The listing builds one solid part. Answer for the finished solid, in the listing's coordinates (mm). Round coordinates to 2 decimals unless told otherwise and drop trailing zeros. Write each loop counter-clockwise with the first axis right and the second up, starting at its lowest first coordinate (ties: lowest second). Pieces come first, ordered by that corner, then holes. Notation, with made-up numbers: M -10,33.25 L 26,33.25 A19 cw 26,61.25 Z; hole C -22.5,-4 d1. An arc over 180 degrees is marked long. Write each question's results on one line, items separated by ' | '.
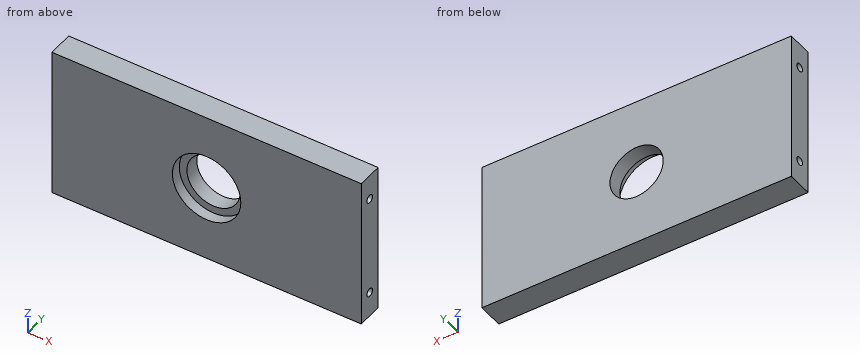
Autodesk Inventor part; units mm, degrees
ref_plane "YZ Plane" through (0, 0, 0) normal (1, 0, 0) x (0, 1, 0)
ref_plane "XZ Plane" through (0, 0, 0) normal (0, 1, 0) x (-1, 0, 0)
ref_plane "XY Plane" through (0, 0, 0) normal (0, 0, 1) x (1, 0, 0)
sketch "スケッチ1" plane through (0, 0, 0) normal (0, 1, 0) x (-1, 0, 0)
  line L0 (61.0285, -30) -> (-61.0285, -30)
  line L1 (-61.0285, -30) -> (-61.0285, 30)
  line L2 (-61.0285, 30) -> (61.0285, 30)
  line L3 (61.0285, 30) -> (61.0285, -30)
  line L4 (61.0285, -30) -> (-61.0285, 30) construction
  line L5 (-61.0285, -30) -> (61.0285, 30) construction
  point P0 (0, 0)
  dimension "d0" = 60
  dimension "d1" = 122.057
extrude "押し出し1" add sketch "スケッチ1" along normal blind 10
sketch "スケッチ2" plane through (0, 0, 0) normal (0, -1, 0) x (1, 0, 0)
  line L0 (-85.4399, 0) -> (85.4399, 0)
  line L1 (0, -42) -> (0, 42)
  circle A0 centre (0, 0) radius 13.5
  dimension "d4" = 27
extrude "押し出し2" cut sketch "スケッチ2" against normal blind 4.1
sketch "スケッチ3" plane through (0, 4.1, 0) normal (0, -1, 0) x (1, 0, 0)
  circle A0 centre (0, 0) radius 10.5
  dimension "d7" = 21
extrude "押し出し4" cut sketch "スケッチ3" against normal blind 10
sketch "スケッチ4" plane through (61.0285, 0, 30) normal (1, 0, 0) x (0, 0, -1)
  line L0 (60, 0) -> (0, 0)
  line L1 (0, 0) -> (0, 10)
  line L2 (60, 0) -> (60, 10)
  point P0 (30, 0)
  point P1 (10, 5)
  point P2 (50, 5)
  dimension "d12" = 5
  dimension "d13" = 10
  dimension "d14" = 10
  dimension "d15" = 5
hole "穴1" at (61.0285, 5, 20) at (61.0285, 5, -20) direction (-1, 0, 0) diameter 3.242 depth 12
sketch "スケッチ5" plane through (-61.0285, 0, -30) normal (-1, 0, 0) x (0, 0, 1)
  line L0 (60, 0) -> (0, 0)
  line L1 (0, 0) -> (0, 10)
  line L2 (60, 0) -> (60, 10)
  point P0 (30, 0)
  point P1 (30, 0)
  point P2 (10, 5)
  point P3 (50, 5)
  dimension "d23" = 5
  dimension "d24" = 10
  dimension "d25" = 10
  dimension "d26" = 5
hole "穴2" at (-61.0285, 5, -20) at (-61.0285, 5, 20) direction (1, 0, 0) diameter 3.242 depth 12
properties part number "Diffbox_plate_main" material "アルミニウム 6061"
1) Section D-D (z = 20) is taken. Determine the outline of the cut face in (x, y), then the cut area to 3 significant figures.
Return value:
outline: M -61.03,0 L 61.03,0 L 61.03,3.38 L 49.03,3.38 L 49.03,6.62 L 61.03,6.62 L 61.03,10 L -61.03,10 L -61.03,6.62 L -49.03,6.62 L -49.03,3.38 L -61.03,3.38 Z | area: 1,140 mm²
2) Find the intervals of material crossed by line 1 (Z direction, x = 58.75, y = 5); line 2 (Y direction, x = -56, z = -20); line 3 (Z direction, x = 0.5, y = 2.5), in increasing order.
Return value:
line 1: -30 to -21.62, -18.38 to 18.38, 21.62 to 30 | line 2: 0 to 3.38, 6.62 to 10 | line 3: -30 to -13.49, 13.49 to 30
3) Section B-B (z = 0) is taken. Determine the outline of the cut face in (x, y).
Return value:
outline: M -61.03,0 L -13.5,0 L -13.5,4.1 L -10.5,4.1 L -10.5,10 L -61.03,10 Z; M 10.5,4.1 L 13.5,4.1 L 13.5,0 L 61.03,0 L 61.03,10 L 10.5,10 Z
4) Section A-A (x = 0) is taken. Determine the outline of the cut face in (y, z), then the cut area to 3 significant figures.
Return value:
outline: M 0,-30 L 10,-30 L 10,-10.5 L 4.1,-10.5 L 4.1,-13.5 L 0,-13.5 Z; M 0,13.5 L 4.1,13.5 L 4.1,10.5 L 10,10.5 L 10,30 L 0,30 Z | area: 365 mm²
5) This flat-tipped pin is pushed along its axis until it touches: pin 1 (1.6 mm diameter, centred on y = 5.5, z = 19.5, fed in from +X). Where does it stop, or does it pass through?
Return value:
pin 1: x = 49.03
6) Section C-C (y = 7.75) is taken. Determine the outline of the cut face in (x, z).
Return value:
outline: M -61.03,-30 L 61.03,-30 L 61.03,30 L -61.03,30 Z; hole C 0,0 d21
